For this review, use the dimensioned drawing (mm, ordinates from the lowest corner) and the shaded views. Give positions to 0.01 mm unless a question says otherwise; leave off trailing zeros. Order: outer loops, then holes, each group sorted by start corner. A loop starts at its lowest first (then second) coordinate and runs counter-clockwise, first axis right, second up. Notation, with made-up numbers: (0, 8) - (6, 8) arc R20 cw to (6, 31) - close; hole circle Ø5 at (-7.75, 17). An arc over 180 degrees is marked (long way). One line per item, written item: value.
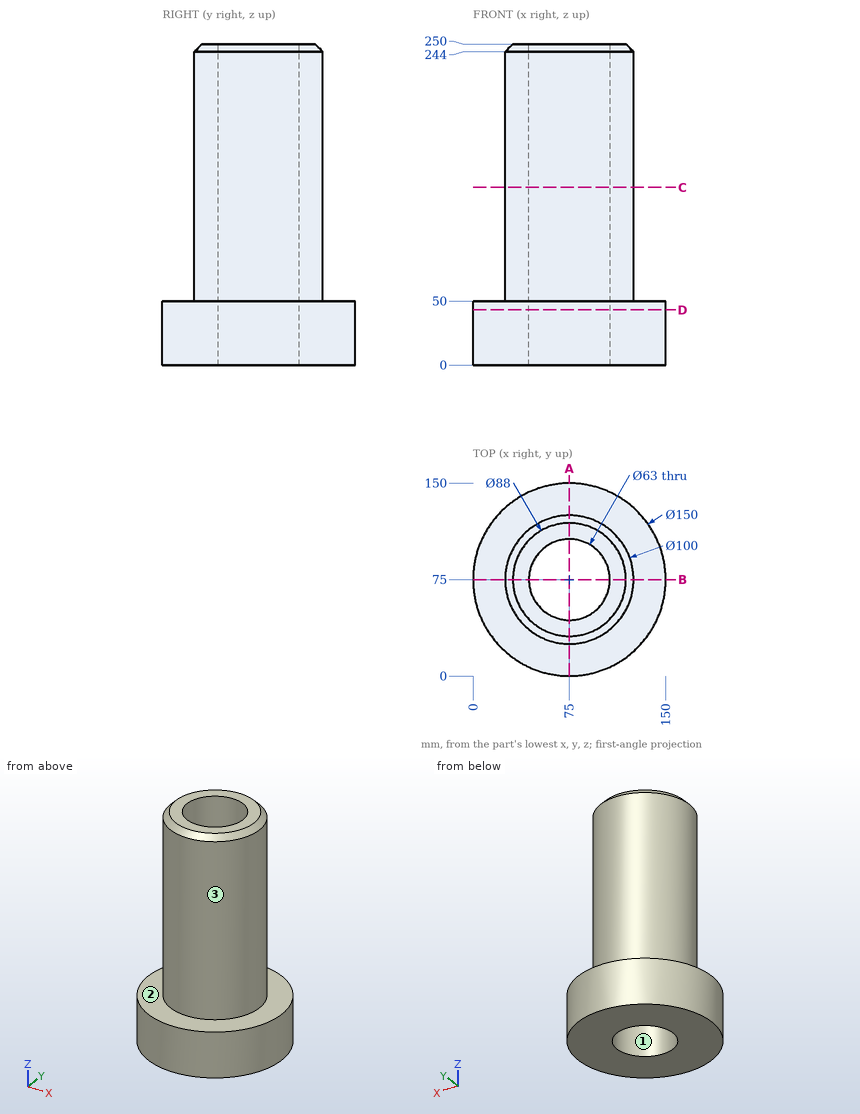
(1) Take a section at A-A (x = 75). Write out the cut boundary in (y, z).
Answers below:
outline: (0, 0) - (43.5, 0) - (43.5, 250) - (31, 250) - (25, 244) - (25, 50) - (0, 50) - close; (106.5, 0) - (150, 0) - (150, 50) - (125, 50) - (125, 244) - (119, 250) - (106.5, 250) - close
(2) For P1, Ø4, axis at x = 59, z = 144.5, coming from the -Y side; P2, Ø12, axis at x = 93.5, y = 67.5, coming from the -Z side; P3, Ø1, axis at y = 45.5, z = 136, coming from the +X side; P4, Ø5, axis at x = 82.5, z = 37.5, coming from the +Y side, all flat-tipped, find the tip position at first contact; note any pin that passes through.
Answers below:
P1: stops at y = 27
P2: passes through
P3: stops at x = 115.73
P4: stops at y = 149.83
(3) Take a section at D-D (z = 43). Write out the cut boundary in (x, y).
Answers below:
outline: circle Ø150 at (75, 75); hole circle Ø63 at (75, 75)
(4) Draft analysis for pull direction Y (two halves, no side actions). For the marked faces 1, 2 and 3, state which applies: pulls with the +Y half, pulls with the -Y half, needs draft (parallel to the pull), parting line crosses it, or undercut.
Answers below:
face 1: undercut
face 2: needs draft
face 3: parting line crosses it
(5) Wall thickness on line 1 (Y direction, x = 75, z = 71); line 2 (X direction, y = 71.5, z = 223); line 3 (X direction, y = 57, z = 116.5): over which ranges is each line inside the solid? List them lowest first. Write a range as from..to.
Answers below:
line 1: y = 25..43.5, 106.5..125
line 2: x = 25.12..43.7, 106.3..124.88
line 3: x = 28.35..49.15, 100.85..121.65
(6) Take a section at C-C (z = 138.5). Write out the cut boundary in (x, y), then the cut area to 3 significant figures.
Answers below:
outline: circle Ø100 at (75, 75); hole circle Ø63 at (75, 75)
area: 4,740 mm^2
